Job drawing, mm, ordinate dimensions from the low corner. One solid piece. A direction names the side the tool comes from. Give positions to 0.01 mm unless a question says otherwise; leave off trailing zeros. Order: outer loops, then holes, each group sorted by start corner. A loop starts at its lowest first (then second) coordinate and runs counter-clockwise, first axis right, second up.
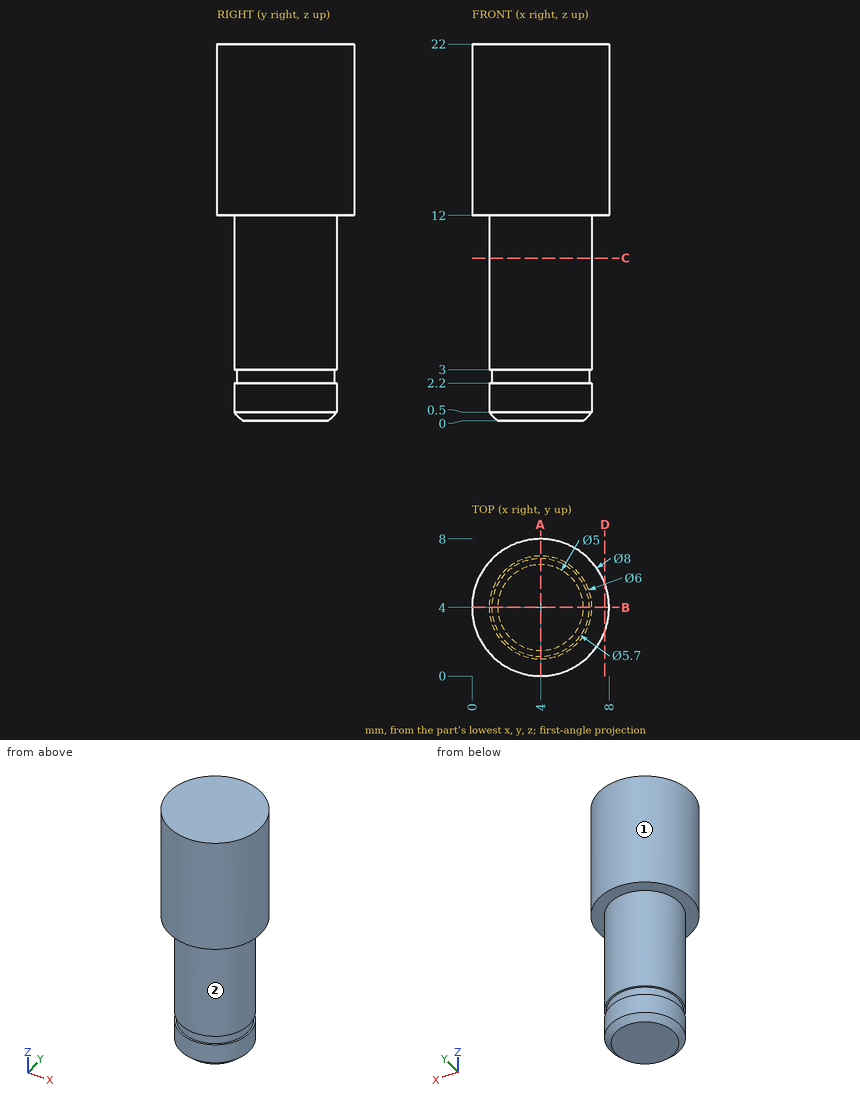
Item 1: Drill centre lines: probe 1 along Z at (x, y) = (0.5, 3.5); probe 2 along X at (y, z) = (6.5, 19.25); probe 3 along Y at (x, z) = (7, 17.25). Where is each one in solid material? Low to high.
Item 2: Band-saw the part on D-D on x = 7.75. List the corners of the cut face in (y, z), plus the area to 3 significant figures.
Item 3: Which spindle directions (+Z, -Z, +X, -X, +Y, -Y) get a long thin tool onto all of the face, cutting with end or side? Do the marked faces 1 and 2. Say none if no direction does.
Item 4: Drop flat-ended pins along their axis: P1, Ø1.5, axis at y = 1, z = 6.5, coming from the +X side; P2, Ø2, axis at x = 5.5, z = 6.5, coming from the +Y side. Give the stop position or say it passes through.
Item 5: Band-saw the part on C-C on z = 9.5. List the corners of the cut face in (x, y).
Item 6: Band-saw the part on A-A on x = 4. List the corners of the cut face in (y, z).
Working result:
1. probe 1: z = 12 to 22
1. probe 2: x = 0.88 to 7.12
1. probe 3: y = 1.35 to 6.65
2. outline: (2.61, 12) - (5.39, 12) - (5.39, 22) - (2.61, 22) - close
2. area: 27.8 mm2
3. face 1: +Z, -Z
3. face 2: -Z
4. P1: stops at x = 5.98
4. P2: stops at y = 6.96
5. outline: circle Ø6 at (4, 4)
6. outline: (0, 12) - (1, 12) - (1, 3) - (1.15, 3) - (1.15, 2.2) - (1, 2.2) - (1, 0.5) - (1.5, 0) - (6.5, 0) - (7, 0.5) - (7, 2.2) - (6.85, 2.2) - (6.85, 3) - (7, 3) - (7, 12) - (8, 12) - (8, 22) - (0, 22) - close
